Verification items for the finished model (mm, model axes). A direction names the side the tool comes from. Coordinates: 2 decimals unless noted, no trailing zeros. Write each loop counter-clockwise with the first axis right and the second up, starting at its lowest first coordinate (ties: lowest second). Pieces come first, ordered by that corner, then holes. Notation, with made-up numbers: (49, 42) -> (97, 42) arc R19 cw to (97, 66) -> close; hole circle Ø1 at (22.5, -28.5). An arc over 180 degrees is marked (long way). Answer in a Markdown table with one row per item.
```python
from build123d import *

# Parameters (mm, degrees)
SKETCH1_W            = 160
SKETCH1_H            = 50
BOSS_EXTRUDE1_DEPTH  = 3
SKETCH2_W            = 160
SKETCH2_H            = 1
CUT_EXTRUDE1_DEPTH   = 1.5
SKETCH3_W            = 5
SKETCH3_H            = 65
BOSS_EXTRUDE2_DEPTH  = 1.5
SKETCH4_W            = 2
SKETCH4_H            = 65
BOSS_EXTRUDE3_DEPTH  = 2
FILLET1_R            = 2
SKETCH5_W            = 160
SKETCH5_H            = 5
BOSS_EXTRUDE4_DEPTH  = 2
SKETCH6_W            = 5
SKETCH6_H            = 160
BOSS_EXTRUDE5_DEPTH  = 2
SKETCH9_W            = 5
SKETCH9_H            = 65
BOSS_EXTRUDE8_DEPTH  = 0.5
SKETCH10_W           = 160
SKETCH10_H           = 3
BOSS_EXTRUDE9_DEPTH  = 5
SKETCH11_W           = 5
SKETCH11_H           = 3
BOSS_EXTRUDE10_DEPTH = 47
SKETCH13_W           = 10
SKETCH13_H           = 46.714659276
BOSS_EXTRUDE11_DEPTH = 5
BOSS_EXTRUDE12_DEPTH = 2
BOSS_EXTRUDE13_DEPTH = 2
BOSS_EXTRUDE14_DEPTH = 0.285341


with BuildPart() as part:
    # Sketch1 → Boss-Extrude1 (new body)
    with BuildSketch(Plane(origin=(0, 0, 0), x_dir=(0, 0, -1), z_dir=(1, 0, 0))):
        Rectangle(SKETCH1_W, SKETCH1_H)
    extrude(amount=BOSS_EXTRUDE1_DEPTH)

    # Sketch2 → Cut-Extrude1 (cut)
    with BuildSketch(Plane(origin=(3, 0, 0), x_dir=(0, 0, -1), z_dir=(1, 0, 0))):
        with Locations((0, -17.5)):
            Rectangle(SKETCH2_W, SKETCH2_H)
        with Locations((0, -6.5)):
            Rectangle(SKETCH2_W, SKETCH2_H)
        with Locations((0, 4.5)):
            Rectangle(SKETCH2_W, SKETCH2_H)
        with Locations((0, 15.5)):
            Rectangle(SKETCH2_W, SKETCH2_H)
    extrude(amount=-CUT_EXTRUDE1_DEPTH, mode=Mode.SUBTRACT)

    # Sketch3 → Boss-Extrude2 (add, symmetric)
    with BuildSketch(Plane(origin=(3, 0, 0), x_dir=(0, 0, -1), z_dir=(1, 0, 0))):
        with Locations((77.5, 7.5)):
            Rectangle(SKETCH3_W, SKETCH3_H)
        with Locations((42.5, 7.5)):
            Rectangle(SKETCH3_W, SKETCH3_H)
        with Locations((-12.5, 7.5)):
            Rectangle(SKETCH3_W, SKETCH3_H)
        with Locations((-67.5, 7.5)):
            Rectangle(SKETCH3_W, SKETCH3_H)
    extrude(amount=BOSS_EXTRUDE2_DEPTH, both=True)

    # Sketch4 → Boss-Extrude3 (add)
    with BuildSketch(Plane(origin=(4.5, 0, 0), x_dir=(0, 0, -1), z_dir=(1, 0, 0))):
        with Locations((44, 7.5)):
            Rectangle(SKETCH4_W, SKETCH4_H)
        with Locations((-11, 7.5)):
            Rectangle(SKETCH4_W, SKETCH4_H)
        with Locations((-66, 7.5)):
            Rectangle(SKETCH4_W, SKETCH4_H)
    extrude(amount=BOSS_EXTRUDE3_DEPTH)

    # Fillet1
    fillet1_edges = [part.edges().sort_by_distance(p)[0] for p in [
        (6.5, 40, -44),
        (6.5, 40, 11),
        (6.5, 40, 66),
    ]]
    fillet(fillet1_edges, radius=FILLET1_R)

    # Sketch5 → Boss-Extrude4 (add)
    with BuildSketch(Plane.ZY):
        with Locations((0, 29.5)):
            Rectangle(SKETCH5_W, SKETCH5_H)
        with Locations((0, 37.5)):
            Rectangle(SKETCH5_W, SKETCH5_H)
    extrude(amount=-BOSS_EXTRUDE4_DEPTH)

    # Sketch6 → Boss-Extrude5 (add)
    with BuildSketch(Plane(origin=(0, 40, 0), x_dir=(1, 0, 0), z_dir=(0, 1, 0))):
        with Locations((2.5, 0)):
            Rectangle(SKETCH6_W, SKETCH6_H)
    extrude(amount=BOSS_EXTRUDE5_DEPTH)

    # Sketch9 → Boss-Extrude8 (add)
    with BuildSketch(Plane(origin=(4.5, 0, 0), x_dir=(0, 0, -1), z_dir=(1, 0, 0))):
        with Locations((77.5, 7.5)):
            Rectangle(SKETCH9_W, SKETCH9_H)
    extrude(amount=BOSS_EXTRUDE8_DEPTH)

    # Sketch10 → Boss-Extrude9 (add)
    with BuildSketch(Plane.ZY):
        with Locations((0, -23.5)):
            Rectangle(SKETCH10_W, SKETCH10_H)
    extrude(amount=BOSS_EXTRUDE9_DEPTH)

    # Sketch11 → Boss-Extrude10 (add)
    with BuildSketch(Plane(origin=(0, -22, 0), x_dir=(1, 0, 0), z_dir=(0, 1, 0))):
        with Locations((-2.5, 78.5)):
            Rectangle(SKETCH11_W, SKETCH11_H)
    extrude(amount=BOSS_EXTRUDE10_DEPTH)

    # Sketch13 → Boss-Extrude11 (add)
    with BuildSketch(Plane.ZY):
        with Locations((80, 1.357329638)):
            Rectangle(SKETCH13_W, SKETCH13_H)
    extrude(amount=BOSS_EXTRUDE11_DEPTH)

    # Sketch14 → Boss-Extrude12 (add)
    with BuildSketch(Plane(origin=(2, 0, 0), x_dir=(0, 0, -1), z_dir=(1, 0, 0))):
        Polygon((75, 40), (75, 35), (67, 40), align=None)
    extrude(amount=BOSS_EXTRUDE12_DEPTH)

    # Sketch15 → Boss-Extrude13 (add)
    with BuildSketch(Plane(origin=(3, 0, 0), x_dir=(0, 0, -1), z_dir=(1, 0, 0))):
        Polygon((75, 25), (45, 25), (45, 20), (49, 21.77425237), (71, 21.77425237), (75, 20), align=None)
    extrude(amount=BOSS_EXTRUDE13_DEPTH)

    # Sketch16 → Boss-Extrude14 (add)
    with BuildSketch(Plane(origin=(0, 24.714659276, 0), x_dir=(1, 0, 0), z_dir=(0, 1, 0))):
        Polygon((0, -75), (-5, -75), (-5, -85), (0, -85), (0, -80), align=None)
    extrude(amount=BOSS_EXTRUDE14_DEPTH)


solid = part.part
```
1. Access from +Z, -Z, +X, -X, +Y, -Y to the whole of each face (thin tool, end or side, straight path). Record for faces 4 (the face through (3, 21, 75)), 5 (the face through (3, -1, -15)), 6 (the face through (2, 38, 40)).
Findings below:
| item | result |
|---|---|
| face 4 | +Z, +X, -Y |
| face 5 | +X, -Y |
| face 6 | +X |
2. Sectioned sample at A-A, the plane z = 17.5. Count the separate pieces of the cut face and the enclosed holes in it, and give its area (3 significant figures).
Findings below:
| item | result |
|---|---|
| separate pieces | 3 |
| enclosed holes | 0 |
| area | 189 mm² |
3. Release check for a two-part mould opening along Z. For faces 1 (the face through (1, 39, 80)), 2 (the face through (2, 30, -15)), 3 (the face through (1.5, 34, 13)) record: released by +Z, released by -Z, zero draft, split by the parting line, or undercut.
Findings below:
| item | result |
|---|---|
| face 1 | released by +Z |
| face 2 | undercut |
| face 3 | zero draft |
4. Sectioned sample at B-B, the plane y = 30. Record the cut outline in (x, z), and give its area (4 significant figures).
Findings below:
| item | result |
|---|---|
| outline | (0, -80) -> (5, -80) -> (5, -75) -> (2, -75) -> (2, -45) -> (6.5, -45) -> (6.5, -43) -> (4.5, -43) -> (4.5, -40) -> (2, -40) -> (2, 10) -> (6.5, 10) -> (6.5, 12) -> (4.5, 12) -> (4.5, 15) -> (2, 15) -> (2, 65) -> (6.5, 65) -> (6.5, 67) -> (4.5, 67) -> (4.5, 70) -> (2, 70) -> (2, 80) -> (0, 80) -> close |
| area | 384.5 mm² |
5. Go/stop test with flat-tipped pins: pin 1 (12 mm diameter, centred on y = -1.5, z = 3.5, fed in from +X); pin 2 (1.5 mm diameter, centred on y = 12.5, z = 68, fed in from +X); pin 3 (0.8 mm diameter, centred on y = -6.5, z = -55.5, fed in from +X). Record where each tip stops, or that it passes through.
Findings below:
| item | result |
|---|---|
| pin 1 | stops at x = 3 |
| pin 2 | stops at x = 4.5 |
| pin 3 | stops at x = 1.5 |
6. Sectioned sample at C-C, the plane x = -3. Record the cut outline in (y, z).
Findings below:
| item | result |
|---|---|
| outline | (-25, -80) -> (25, -80) -> (25, -77) -> (-22, -77) -> (-22, 75) -> (25, 75) -> (25, 85) -> (-22, 85) -> (-22, 80) -> (-25, 80) -> close |
7. Material ranges on probe 1 along Z at (x, y) = (5.5, -13.5); probe 2 along Z at (x, y) = (4.75, 8.5); probe 3 along Z at (x, y) = (-3.5, 17), recorded low to high. Write a range as from..to.
Findings below:
| item | result |
|---|---|
| probe 1 | z = -45..-43, 10..12, 65..67 |
| probe 2 | z = -80..-75, -45..-43, 10..12, 65..67 |
| probe 3 | z = -80..-77, 75..85 |
